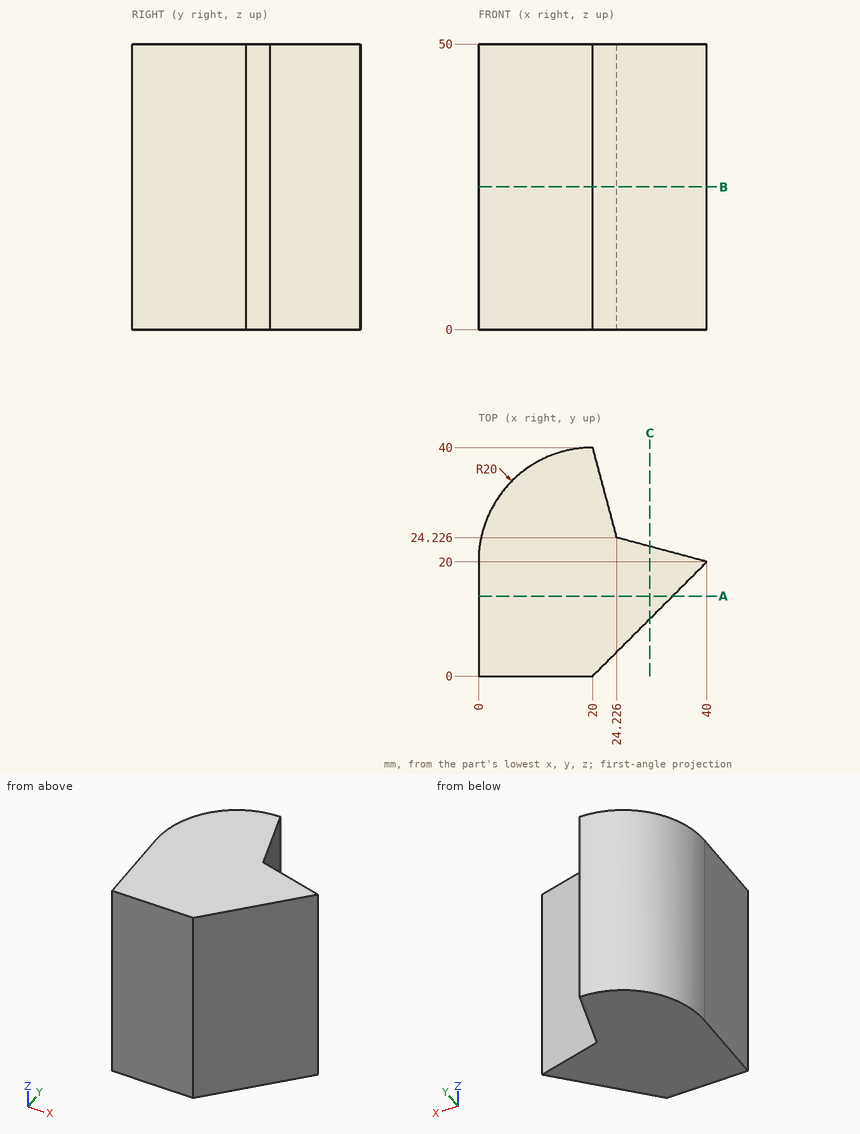
Input: dimensioned drawing with shaded views. Units: mm. Origin: part minimum x, y, z. Coordinates: 2 decimals unless noted, no trailing zeros. Order: outer loops, then holes, each group sorted by start corner. A loop starts at its lowest first (then second) coordinate and runs counter-clockwise, first axis right, second up. Notation, with made-up numbers: (77, 81.5) - (114, 81.5) arc R23 ccw to (114, 111.5) - close; hole circle Ø5 at (18.5, 30.5). An arc over 180 degrees is marked (long way). One line per item, written item: value.
1) Ray query, line 1 (X direction, y = 26, z = 27.5); line 2 (Y direction, x = 10.5, z = 43.5); line 3 (Y direction, x = 13, z = 40) (1 decimal). Return the intervals inside material, ascending. Write a range as [from, to].
Computed values:
line 1: x = [0.92, 23.75]
line 2: y = [0, 37.6]
line 3: y = [0, 38.7]
2) Cut plane C-C on x = 30. Output: boundary loops of the cut face in (y, z), plus the area to 3 significant figures.
Computed values:
outline: (10, 0) - (22.68, 0) - (22.68, 50) - (10, 50) - close
area: 634 mm^2
3) Cut plane B-B on z = 25. Output: boundary loops of the cut face in (x, y), plus the area to 3 significant figures.
Computed values:
outline: (0, 0) - (20, 0) - (40, 20) - (24.23, 24.23) - (20, 40) arc R20 ccw to (0, 20) - close
area: 999 mm^2
4) Contact query for flat-ended pins moving along their axis: pin 1 (4 mm diameter, centred on y = 35, z = 44, fed in from +X) (1 decimal); pin 2 (10 mm diameter, centred on x = 27, z = 39, fed in from -Y); pin 3 (3 mm diameter, centred on y = 17, z = 20, fed in from +X). Output: stop coordinate, or through.
Computed values:
pin 1: stops at x = 21.9
pin 2: stops at y = 2
pin 3: stops at x = 38.5
5) Cut plane A-A on y = 14. Output: boundary loops of the cut face in (x, z).
Computed values:
outline: (0, 0) - (34, 0) - (34, 50) - (0, 50) - close
